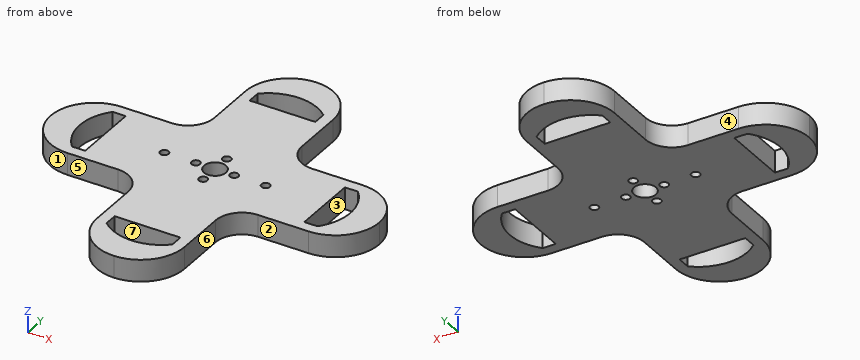
from build123d import *

# Parameters (mm, degrees)
EXTRUDE_1_DEPTH          = 5
CUT_EXTRUDE_1_DEPTH      = 54.268189382
FILLET_1_R               = 10
FILLET_2_R               = 6
SCALE_1_SCALE            = 1.6
CUT_EXTRUDE_2_DEPTH      = 86.229103011
CUT_EXTRUDE_2_DEPTH_BACK = 86.229103011
SKETCH_3_R               = 4
SKETCH_3_R_2             = 1.55


with BuildPart() as part:
    # 草图1 → 凸台-拉伸1 (new body)
    with BuildSketch(Plane.XY):
        Polygon((-10, 32.5), (-10, 10), (-37.5, 10), (-37.5, -10), (-10, -10), (-10, -37.5), (10, -37.5), (10, -10), (37.5, -10), (37.5, 10), (10, 10), (10, 32.5), (10, 37.5), (0, 37.5), (-10, 37.5), align=None)
    extrude(amount=EXTRUDE_1_DEPTH)

    # 草图2 → 切除-拉伸1 (cut, through all)
    with BuildSketch(Plane.XY.offset(5)):
        with BuildLine():
            Line((7.5, 25), (7.5, 28))
            ThreePointArc((7.5, 28), (0, 30.881947343), (-7.5, 28))
            Line((-7.5, 28), (-7.5, 25))
            Line((-7.5, 25), (7.5, 25))
        make_face()
        with BuildLine():
            ThreePointArc((-28, -7.5), (-30.881947343, 0), (-28, 7.5))
            Line((-28, 7.5), (-25, 7.5))
            Line((-25, 7.5), (-25, -7.5))
            Line((-25, -7.5), (-28, -7.5))
        make_face()
        with BuildLine():
            ThreePointArc((7.5, -28), (0, -30.881947343), (-7.5, -28))
            Line((-7.5, -28), (-7.5, -25))
            Line((-7.5, -25), (7.5, -25))
            Line((7.5, -25), (7.5, -28))
        make_face()
        with BuildLine():
            ThreePointArc((28, 7.5), (30.881947343, 0), (28, -7.5))
            Line((28, -7.5), (25, -7.5))
            Line((25, -7.5), (25, 7.5))
            Line((25, 7.5), (28, 7.5))
        make_face()
    extrude(amount=-CUT_EXTRUDE_1_DEPTH, mode=Mode.SUBTRACT)

    # 圆角1
    fillet_1_edges = [part.edges().sort_by_distance(p)[0] for p in [
        (-37.5, 10, 2.5),
        (-37.5, -10, 2.5),
        (-10, -37.5, 2.5),
        (10, -37.5, 2.5),
        (37.5, -10, 2.5),
        (37.5, 10, 2.5),
        (10, 37.5, 2.5),
        (-10, 37.5, 2.5),
    ]]
    fillet(fillet_1_edges, radius=FILLET_1_R - 0.0001)  # a hair under: the kernel refuses the full size

    # 圆角2
    fillet_2_edges = [part.edges().sort_by_distance(p)[0] for p in [
        (10, 10, 2.5),
        (10, -10, 2.5),
        (-10, -10, 2.5),
        (-10, 10, 2.5),
    ]]
    fillet(fillet_2_edges, radius=FILLET_2_R)


with BuildPart() as part_1:
    # 缩放比例1: scaled about (0, 0, 2.5)
    add(part.part.scale(SCALE_1_SCALE).moved(Location((0, 0, -1.5))))

    # 草图3 → 切除-拉伸2 (cut, two sides: drawn at the far end of the back side and taken through both)
    with BuildSketch(Plane.XY.offset(6.5).offset(-CUT_EXTRUDE_2_DEPTH_BACK)):
        Circle(SKETCH_3_R)
        with Locations((-7, 0)):
            Circle(SKETCH_3_R_2)
        with Locations((7, 0)):
            Circle(SKETCH_3_R_2)
        with Locations((0, 7)):
            Circle(SKETCH_3_R_2)
        with Locations((0, -7)):
            Circle(SKETCH_3_R_2)
        with Locations((-18.5, 0)):
            Circle(SKETCH_3_R_2)
        with Locations((18.5, 0)):
            Circle(SKETCH_3_R_2)
    extrude(amount=CUT_EXTRUDE_2_DEPTH + CUT_EXTRUDE_2_DEPTH_BACK, mode=Mode.SUBTRACT)


solid = part_1.part
Model file for the job. Use its own axes, mm. Face numbers are marked on the shaded views. A direction names the side the tool comes from. Give positions to 0.01 mm unless a question says otherwise; leave off trailing zeros. Order: outer loops, then holes, each group sorted by start corner. A loop starts at its lowest first (then second) coordinate and runs counter-clockwise, first axis right, second up. Notation, with made-up numbers: (34.25, 24) - (48.25, 24) arc R34 ccw to (48.25, 54) - close; hole circle Ø8 at (53.5, -5). An arc over 180 degrees is marked (long way). Return JSON: item names as keys, results as strings.
1) Cut at C-C, the plane z = 1. Count the separate pieces of the cut face and the enclosed holes in it, plus the area to 3 significant figures.
Geometry says:
{"separate pieces": "1", "enclosed holes": "11", "area": "5,440 mm²"}
2) Cut at D-D, the plane y = 28. Give the cut face in (x, z).
Geometry says:
{"outline": "(-16, -1.5) - (16, -1.5) - (16, 6.5) - (-16, 6.5) - close"}
3) Flat gauge pins, fed straight in: P1, Ø4, axis at y = 35.5, z = 4.5, coming from the -X side; P2, Ø2.5, axis at x = 43.5, z = 2, coming from the -Y side; P3, Ø2.5, axis at x = 0, y = 7, coming from the -Z side; P4, Ø4, axis at x = -35, z = 0.5, coming from the +Y side. Where does each tip first touch, or does it go through?
Geometry says:
{"P1": "x = -16", "P2": "y = -16", "P3": "through", "P4": "y = 16"}
4) Cut at A-A, the plane y = 7. Give the cut face in (x, z).
Geometry says:
{"outline": "(-58.39, -1.5) - (-47.99, -1.5) - (-47.99, 6.5) - (-58.39, 6.5) - close; (-40, -1.5) - (-1.55, -1.5) - (-1.55, 6.5) - (-40, 6.5) - close; (1.55, -1.5) - (40, -1.5) - (40, 6.5) - (1.55, 6.5) - close; (47.99, -1.5) - (58.39, -1.5) - (58.39, 6.5) - (47.99, 6.5) - close"}
5) Cut at B-B, the plane x = 18.5. Give the cut face in (y, z), plus the area to 3 significant figures.
Geometry says:
{"outline": "(-19.14, -1.5) - (-1.55, -1.5) - (-1.55, 6.5) - (-19.14, 6.5) - close; (1.55, -1.5) - (19.14, -1.5) - (19.14, 6.5) - (1.55, 6.5) - close", "area": "281 mm²"}
6) 3-axis set-ups, long thin cutter, end or side, ignore diameter. For the marked faces 4, 5, 6 and 7: which of +Z, -Z, +X, -X, +Y, -Y reach the whole face in a straight line?
Geometry says:
{"face 4": "+Z, -Z, -X, +Y", "face 5": "+Z, -Z, -X, -Y", "face 6": "+Z, -Z, +X, -Y", "face 7": "+Z, -Z"}
7) Pull direction X, two halves, no side cores. Call the marked faces 1, 2 and 3: pulls with the +X half, pulls with the -X half, needs draft (parallel to the pull), parting line crosses it, or undercut.
Geometry says:
{"face 1": "pulls with the -X half", "face 2": "needs draft", "face 3": "undercut"}
8) Probe line 1 (Y direction, x = 0, z = 0); line 2 (Y direction, x = 11, z = 2.5); line 3 (X direction, y = -41, z = 5). List the from-to ranges inside material, lowest first. Write a range as from..to.
Geometry says:
{"line 1": "-60..-49.41, -40..-8.55, -5.45..-4, 4..5.45, 8.55..40, 49.41..60", "line 2": "-55.62..-45.64, -40..40, 45.64..55.62", "line 3": "-16..-12, 12..16"}
